Design review of the part built by this model. Coordinates are the model's own, in mm. A direction names the side the tool comes from. Give positions to 0.01 mm unless a question says otherwise; leave off trailing zeros. Loops run counter-clockwise (first coordinate to the right, second up) from the corner with the lowest first, then second, coordinate; pieces in that order, holes last. Notation, with made-up numbers: M 19.25,10 L 28.25,10 A27 ccw 28.25,42 Z; hole C -36,-2 d9. An arc over 180 degrees is marked long. Use one line per item in the form item = value. Start each with the question number.
from build123d import *
from build123d.topology import SkipClean

# Parameters (mm, degrees)
SKETCH1_R           = 10.5
SKETCH1_R_2         = 8.6
BOSS_EXTRUDE1_DEPTH = 3.5
BOSS_EXTRUDE2_DEPTH = 1.25
BOSS_EXTRUDE3_START = 17.2
BOSS_EXTRUDE3_DEPTH = 1.25
BOSS_EXTRUDE4_START = 0.5
SKETCH3_R           = 10.5
BOSS_EXTRUDE4_DEPTH = 0.5
SKETCH5_R           = 3.25
BOSS_EXTRUDE5_DEPTH = 6
FILLET2_R           = 0.75
CUT_EXTRUDE1_DEPTH  = 5.5
FILLET1_R           = 0.25
SKETCH7_R           = 2.625
CUT_EXTRUDE2_DEPTH  = 2.5
CUT_EXTRUDE3_DEPTH  = 0.25
SKETCH11_R          = 2.5
BOSS_EXTRUDE6_DEPTH = 5
CUT_EXTRUDE4_START  = 5
CUT_EXTRUDE4_DEPTH  = 4.5
CHAMFER2_SIZE       = 0.25
FILLET3_R           = 5


with BuildPart() as part:
    # Sketch1 → Boss-Extrude1 (new body)
    with BuildSketch(Plane(origin=(0, 0, 0), x_dir=(1, 0, 0), z_dir=(0, 1, 0))):
        with Locations(Location((0, 0, 0), (0, 0, 270))):
            Circle(SKETCH1_R)
        with Locations(Location((0, 0, 0), (0, 0, 270))):
            Circle(SKETCH1_R_2, mode=Mode.SUBTRACT)
    extrude(amount=-BOSS_EXTRUDE1_DEPTH)

    # Sketch2 → Boss-Extrude2 (add)
    with BuildSketch(Plane(origin=(0, 0, 8.6), x_dir=(-1, 0, 0), z_dir=(0, 0, -1))):
        Polygon((0.4, -2.9), (-0.4, -2.9), (-0.4, -1), (-1.4, 0), (1.4, 0), (0.4, -1), align=None)
    extrude(amount=BOSS_EXTRUDE2_DEPTH)

    # Sketch2<2> → Boss-Extrude3 (add)
    with BuildSketch(Plane(origin=(0, 0, 8.6), x_dir=(-1, 0, 0), z_dir=(0, 0, -1)).offset(BOSS_EXTRUDE3_START)):
        Polygon((0.4, -2.9), (-0.4, -2.9), (-0.4, -1), (-1.4, 0), (1.4, 0), (0.4, -1), align=None)
    extrude(amount=-BOSS_EXTRUDE3_DEPTH)

    # Sketch3 → Boss-Extrude4 (add)
    with BuildSketch(Plane(origin=(0, 0, 0), x_dir=(1, 0, 0), z_dir=(0, 1, 0)).offset(BOSS_EXTRUDE4_START)):
        with Locations(Location((0, 0, 0), (0, 0, 270))):
            Circle(SKETCH3_R)
    extrude(amount=-BOSS_EXTRUDE4_DEPTH)

    # Sketch5 → Boss-Extrude5 (add)
    with BuildSketch(Plane.XZ):
        with Locations(Location((0, 0, 0), (0, 0, 90))):
            Circle(SKETCH5_R)
    extrude(amount=BOSS_EXTRUDE5_DEPTH)

    # Fillet2
    fillet2_edges = [part.edges().sort_by_distance(p)[0] for p in [
        (0, 0, -3.25),
    ]]
    fillet(fillet2_edges, radius=FILLET2_R)

    # Sketch4 → Cut-Extrude1 (cut)
    with BuildSketch(Plane(origin=(0, 0.5, 0), x_dir=(1, 0, 0), z_dir=(0, 1, 0))):
        with BuildLine():
            Line((-1.469693846, 2.175), (1.469693846, 2.175))
            ThreePointArc((1.469693846, 2.175), (0, -2.625), (-1.469693846, 2.175))
        make_face()
    extrude(amount=-CUT_EXTRUDE1_DEPTH, mode=Mode.SUBTRACT)

    # Fillet1
    fillet1_edges = [part.edges().sort_by_distance(p)[0] for p in [
        (-0.4, -2.9, 7.970346319),
        (0.4, -2.9, 7.970346319),
        (-0.4, -2.9, -7.970346319),
        (0.4, -2.9, -7.970346319),
    ]]
    fillet(fillet1_edges, radius=FILLET1_R)

    # Sketch7 → Cut-Extrude2 (cut)
    with SkipClean():  # the faces are left unmerged after this step: merging them gives an invalid solid
        with BuildSketch(Plane(origin=(0, 0.5, 0), x_dir=(1, 0, 0), z_dir=(0, 1, 0))):
            with Locations(Location((0, 0, 0), (0, 0, 270))):
                Circle(SKETCH7_R)
        extrude(amount=-CUT_EXTRUDE2_DEPTH, mode=Mode.SUBTRACT)

    # Sketch9 → Cut-Extrude3 (cut)
    with SkipClean():  # the faces are left unmerged after this step: merging them gives an invalid solid
        with BuildSketch(Plane(origin=(0, 0.5, 0), x_dir=(1, 0, 0), z_dir=(0, 1, 0))):
            with BuildLine():
                Line((-0.5, 3.7), (-0.5, 13.7))
                ThreePointArc((-0.5, 13.7), (0, 14.2), (0.5, 13.7))
                Line((0.5, 13.7), (0.5, 3.7))
                ThreePointArc((0.5, 3.7), (0, 3.2), (-0.5, 3.7))
            make_face()
        extrude(amount=-CUT_EXTRUDE3_DEPTH, mode=Mode.SUBTRACT)

    # Sketch11 → Boss-Extrude6 (add)
    with SkipClean():  # the faces are left unmerged after this step: merging them gives an invalid solid
        with BuildSketch(Plane.XZ.offset(6)):
            with Locations(Location((0, 0, 0), (0, 0, 270))):
                Circle(SKETCH11_R)
        extrude(amount=BOSS_EXTRUDE6_DEPTH)

    # Sketch10 → Cut-Extrude4 (cut)
    with SkipClean():  # the faces are left unmerged after this step: merging them gives an invalid solid
        with BuildSketch(Plane.XZ.offset(6).offset(CUT_EXTRUDE4_START)):
            Polygon((1.804219591, 0), (0.902109796, 1.5625), (-0.902109796, 1.5625), (-1.804219591, 0), (-0.902109796, -1.5625), (0.902109796, -1.5625), align=None)
        extrude(amount=-CUT_EXTRUDE4_DEPTH, mode=Mode.SUBTRACT)

    # Chamfer2
    chamfer2_edges = [part.edges().sort_by_distance(p)[0] for p in [
        (-1.353164693, -11, -0.78125),
        (-1.353164693, -11, 0.78125),
        (0, -11, 1.5625),
        (1.353164693, -11, 0.78125),
        (1.353164693, -11, -0.78125),
        (0, -11, -1.5625),
    ]]
    chamfer(chamfer2_edges, length=CHAMFER2_SIZE)

    # Fillet3
    # the kernel refuses this fillet: 5 mm, written as the material it adds along each edge
    with BuildSketch(Plane(origin=(0, -6, 0), x_dir=(0, 0, -1), z_dir=(-1, 0, 0))) as fillet3_piece_1:
        with BuildLine():
            CenterArc((7.5, 2.633913438), FILLET3_R, 180, 31.788330617)
            Line((3.25, 0), (3.165, -0.052678269))
            ThreePointArc((3.165, -0.052678269), (2.875, -0.1), (2.5, -0.1))
            Line((2.5, -0.1), (2.4, 0))
            Line((2.4, 0), (2.4, 2.633913438))
            Line((2.4, 2.633913438), (2.5, 2.633913438))
        make_face()
    revolve(axis=Axis((0, -6, 0), (0, -1, 0)))


solid = part.part
Q1. For faces 4 (the cylindrical face through (3.2, -1.5, 10)), 5 (the flat face through (1.35, -8.65, -0.79)), 6 (the flat face through (0, -3, -2.175)), 7 (the flat face through (0, 0.25, -7)), list the 3-axis set-ups (+Z, -Z, +X, -X, +Y, -Y) from which the entire face can be reached by the end or side of a thin tool; tool diameter is ignored.
Q2. Take a section at A-A on z = 5. Give the boundary of the cut face in (x, y), plus the area to 3 significant figures.
Q3. Wall thickness on probe 1 along X at (y, z) = (-2.5, 0) (3 decimals); probe 2 along X at (y, z) = (-2.25, -2.5); probe 3 along Y at (x, z) = (-5.25, -3.75): over which ranges is each line inside the solid? List them lowest first.
Q4. The part is to be moulded in two halves that separate along X. For faces 1 (the cylindrical face through (-2.44, -9.8, 0.54)), 2 (the flat face through (0.4, -2, -8)), 3 (the flat face through (0, -11, -2)), say which applies: pulls with the +X half, pulls with the -X half, needs draft (parallel to the pull), parting line crosses it, or undercut.
Q5. Clearance check with flat-ended pins moving along their axes: pin 1 Ø6 at (y, z) = (-0.5, 5) entering from -X; pin 2 Ø2 at (x, y) = (0, -8.5) entering from -Z; pin 3 Ø0.6 at (y, z) = (-1.5, 8) entering from +X; pin 4 Ø3 at (x, y) = (-1.5, -4) entering from -Z. State where each tip first meets the part, or that it passes through.
Response values:
q1.face_4 = +Y, -Y
q1.face_5 = -Y
q1.face_6 = +Y
q1.face_7 = -Z, +Y
q2.outline = M -9.23,-3.5 L -7,-3.5 L -7,0 L 7,0 L 7,-3.5 L 9.23,-3.5 L 9.23,0.5 L -9.23,0.5 Z
q2.area = 24.9 mm^2
q3.probe_1 = -10.5 to -8.6, -3.25 to -2.625, 2.625 to 3.25, 8.6 to 10.5
q3.probe_2 = -10.2 to -8.23, -2.08 to 2.08, 8.23 to 10.2
q3.probe_3 = 0 to 0.5
q4.face_1 = parting line crosses it
q4.face_2 = undercut
q4.face_3 = needs draft
q5.pin_1 = -10.31
q5.pin_2 = -2.63
q5.pin_3 = 7.14
q5.pin_4 = -10.5
